from build123d import *

# Parameters (mm, degrees)
EXTRUDE_1_DEPTH          = 4
CUT_EXTRUDE_1_DEPTH      = 50.678969393496885
SKETCH_5_R               = 10
CUT_EXTRUDE_2_DEPTH      = 3.4
SKETCH_6_R               = 0.7
SKETCH_6_R_2             = 0.7000000000000005
CUT_EXTRUDE_3_DEPTH      = 50.24591353604885
SKETCH_8_R               = 4.25
CUT_EXTRUDE_5_DEPTH      = 50.24591353604885
CUT_EXTRUDE_7_DEPTH      = 50.193495504995376
CUT_EXTRUDE_7_DEPTH_BACK = 50.193495504995376
FILLET_1_R               = 1
CHAMFER_1_SIZE           = 1
CHAMFER_3_SIZE           = 1


with BuildPart() as part:
    # 草图1 → 凸台-拉伸1 (new, symmetric)
    with BuildSketch(Plane.XY):
        with BuildLine():
            Line((0.9523809523809523, 9.954545219222322), (42.57142857142857, 5.972727131533395))
            ThreePointArc((42.57142857142857, 5.972727131533395), (48, 0), (42.57142857142857, -5.972727131533395))
            Line((42.57142857142857, -5.972727131533395), (0.9523809523809523, -9.954545219222322))
            ThreePointArc((0.9523809523809523, -9.954545219222322), (-10.000000000000002, 1.22e-15), (0.9523809523809523, 9.954545219222322))
        make_face()
    extrude(amount=EXTRUDE_1_DEPTH, both=True)

    # 草图3 → 切除-拉伸1 (cut, through all)
    with BuildSketch(Plane.XY.offset(4)):
        with BuildLine():
            Line((38, 2.55), (42, 2.55))
            ThreePointArc((42, 2.55), (44.55, 0), (42, -2.55))
            Line((42, -2.55), (38, -2.55))
            ThreePointArc((38, -2.55), (35.45, 3.1e-16), (38, 2.55))
        make_face()
    extrude(amount=-CUT_EXTRUDE_1_DEPTH, mode=Mode.SUBTRACT)

    # 草图5 → 切除-拉伸2 (cut)
    with BuildSketch(Plane.XY.offset(4)):
        Circle(SKETCH_5_R)
    cut_extrude_2 = extrude(amount=-CUT_EXTRUDE_2_DEPTH, mode=Mode.SUBTRACT)

    # 镜向7: 切除-拉伸2 across plane
    add(cut_extrude_2.mirror(Plane.XY), mode=Mode.SUBTRACT)

    # 草图6 → 切除-拉伸3 (cut, through all)
    with BuildSketch(Plane.XY.offset(0.6000000000000003)):
        with Locations((0, 7)):
            Circle(SKETCH_6_R)
        with Locations((0, -7)):
            Circle(SKETCH_6_R)
        with Locations((7, -1.8e-15)):
            Circle(SKETCH_6_R_2)
        with Locations((-7, -1.8e-15)):
            Circle(SKETCH_6_R_2)
    extrude(amount=-CUT_EXTRUDE_3_DEPTH, mode=Mode.SUBTRACT)

    # 草图8 → 切除-拉伸5 (cut, through all)
    with BuildSketch(Plane.XY.offset(0.6000000000000003)):
        Circle(SKETCH_8_R)
    extrude(amount=-CUT_EXTRUDE_5_DEPTH, mode=Mode.SUBTRACT)

    # 草图10 → 切除-拉伸7 (cut, two sides: drawn at the far end of the back side and taken through both)
    with BuildSketch(Plane(origin=(0, 0, 0), x_dir=(1, 0, 0), z_dir=(0, 1, 0)).offset(-CUT_EXTRUDE_7_DEPTH_BACK)):
        Polygon((0.9523809523809523, 1.6000000000000003), (0.9523809523809523, 4), (20.952380952380953, 4.000000000000003), align=None)
        Polygon((0.9523809523809523, -2.4), (20.95238095238096, 6.07e-15), (48.00000000000001, 6.07e-15), (48.00000000000001, -4), (0.952380952380952, -4), align=None)
    extrude(amount=CUT_EXTRUDE_7_DEPTH + CUT_EXTRUDE_7_DEPTH_BACK, mode=Mode.SUBTRACT)

    # 圆角1
    fillet_1_edges = [part.edges().sort_by_distance(p)[0] for p in [
        (0.9523809523809526, 9.954545219222322, -1.0999999999999996),
        (0.9523809523809524, -9.954545219222322, -1.0999999999999996),
        (0.9523809523809526, 9.954545219222322, 1.5),
        (0.9523809523809524, -9.954545219222322, 1.5),
    ]]
    fillet(fillet_1_edges, radius=FILLET_1_R)

    # 倒角1
    chamfer_1_edges = [part.edges().sort_by_distance(p)[0] for p in [
        (31.761904761904763, 7.006906428907978, -4),
        (48, 1.33e-15, -4),
        (31.761904761904763, -7.006906428907978, -4),
        (48, 1.33e-15, -6.07e-15),
        (31.761904761904763, -7.006906428907977, -6.07e-15),
        (31.761904761904766, 7.006906428907978, -6.07e-15),
    ]]
    chamfer(chamfer_1_edges, length=CHAMFER_1_SIZE)

    # 倒角3
    # the kernel refuses this chamfer: 1 mm, written as the material it adds along each edge
    with BuildSketch(Plane(origin=(0, 0, -0.6000000000000001), x_dir=(0.6502681863563081, -0.7597047359421143, 0), z_dir=(-0.7597047359421143, -0.6502681863563081, 0))) as chamfer_3_piece_1:
        Polygon((10, -CHAMFER_3_SIZE), (9.999999999999998 - CHAMFER_3_SIZE, -2e-16), (9.999999999999998, 0), align=None)
    revolve(axis=Axis((0, 0, -0.6000000000000001), (0, 2e-17, 1)), revolution_arc=98.87634994501913)
    with BuildSketch(Plane(origin=(7.1529500499193945, 8.356752095363253, -0.6000000000000001), x_dir=(0.45453302112340566, -0.8907298876249914, 0), z_dir=(-0.8907298876249914, -0.45453302112340566, 0))) as chamfer_3_piece_2_section:
        Polygon((1.0000000000000004, -CHAMFER_3_SIZE), (1.0000000000000004 + CHAMFER_3_SIZE, 0), (1.0000000000000004, 0), align=None)
    chamfer_3_piece_2 = revolve(axis=Axis((7.1529500499193945, 8.356752095363253, -0.6000000000000001), (0, 0, 1)), revolution_arc=292.40328295994874, mode=Mode.PRIVATE)
    chamfer_3_piece_2 = split(chamfer_3_piece_2, bisect_by=Plane(origin=(6.105913725446883, 9.461491408882363, -0.9544569882762437), z_dir=(-0.09523809523809522, -0.995454521922232, 0)), keep=Keep.TOP, mode=Mode.PRIVATE)
    add(chamfer_3_piece_2)
    with BuildSketch(Plane(origin=(7.152950049919392, -8.356752095363255, -0.6000000000000001), x_dir=(0.4545330211234144, 0.8907298876249867, 0), z_dir=(-0.8907298876249867, 0.4545330211234144, 0))) as chamfer_3_piece_3_section:
        Polygon((1.0000000000000002 + CHAMFER_3_SIZE, 0), (0.9999999999999994, CHAMFER_3_SIZE), (1.0000000000000002, 0), align=None)
    chamfer_3_piece_3 = revolve(axis=Axis((7.152950049919392, -8.356752095363255, -0.6000000000000001), (0, 0, -1)), revolution_arc=292.40328295994846, mode=Mode.PRIVATE)
    chamfer_3_piece_3 = split(chamfer_3_piece_3, bisect_by=Plane(origin=(6.105912616149652, -9.46149151501213, -0.9544569410111913), z_dir=(-0.09523809523809522, 0.995454521922232, 0)), keep=Keep.TOP, mode=Mode.PRIVATE)
    add(chamfer_3_piece_3)


solid = part.part
Geometry check sheet. Reference: the model listing, model coordinates, mm. A direction names the side the tool comes from. Give positions to 0.01 mm unless a question says otherwise; leave off trailing zeros. Order: outer loops, then holes, each group sorted by start corner. A loop starts at its lowest first (then second) coordinate and runs counter-clockwise, first axis right, second up.
1. Depth check by flat-ended pin: pin 1 (4 mm diameter, centred on x = -4, y = 7, fed in from -Z); pin 2 (3 mm diameter, centred on x = 40, z = -2, fed in from -Y); pin 3 (11.5 mm diameter, centred on x = 33.5, y = -1.5, fed in from +Z). Enter the tip coordinate at first touch or a pass-through.
Completed:
pin 1: stops at z = -0.6
pin 2: stops at y = -6.36
pin 3: stops at z = 0
2. Draft check along Y on faces 1 (the face through (34.3, 6.27, -0.51)), 2 (the face through (48, 0, -2)), 3 (the face through (6.3, 0, 0)). Enter one of: pulls with the +Y half, pulls with the -Y half, needs draft (parallel to the pull), parting line crosses it, or undercut.
Completed:
face 1: pulls with the +Y half
face 2: parting line crosses it
face 3: undercut
3. Access from +Z, -Z, +X, -X, +Y, -Y to the whole of each face (thin tool, end or side, straight path). Record for faces 4 (the face through (10, 0, -2)), 5 (the face through (40, -2.55, -2)), 6 (the face through (31, 0, 0)).
Completed:
face 4: -Z, -X
face 5: +Z, -Z
face 6: +Z, +X, +Y, -Y
4. Sectioned sample at B-B (x = -7). Record the boundary of the cut face in (y, z).
Completed:
outline: (-7.14, -0.6) - (-0.7, -0.6) - (-0.7, 0.6) - (-7.14, 0.6) - close; (0.7, -0.6) - (7.14, -0.6) - (7.14, 0.6) - (0.7, 0.6) - close
5. Sectioned sample at A-A (x = 0). Record the boundary of the cut face in (y, z), then the cut area to 3 significant figures.
Completed:
outline: (-10, -0.6) - (-7.7, -0.6) - (-7.7, 0.6) - (-10, 0.6) - close; (-6.3, -0.6) - (-4.25, -0.6) - (-4.25, 0.6) - (-6.3, 0.6) - close; (4.25, -0.6) - (6.3, -0.6) - (6.3, 0.6) - (4.25, 0.6) - close; (7.7, -0.6) - (10, -0.6) - (10, 0.6) - (7.7, 0.6) - close
area: 10.4 mm2
6. Scan lines: line 1 (Y direction, x = 0, z = 0.3); line 2 (Y direction, x = 0.5, z = 0.45); line 3 (Z direction, x = 23.5, y = 0.25). Record each from-to range of solid material in increasing order.
Completed:
line 1: y = -10 to -7.7, -6.3 to -4.25, 4.25 to 6.3, 7.7 to 10
line 2: y = -9.99 to -7.49, -6.51 to -4.22, 4.22 to 6.51, 7.49 to 9.99
line 3: z = -4 to 0
7. Sectioned sample at C-C (y = 0). State how many separate pieces and enclosed holes the cut face has, then the cut area to 3 significant figures.
Completed:
separate pieces: 5
enclosed holes: 0
area: 126 mm2
8. Sectioned sample at D-D (x = 15). Record the boundary of the cut face in (y, z).
Completed:
outline: (-8.61, -3) - (-8.32, -3.29) - (8.32, -3.29) - (8.61, -3) - (8.61, 0.71) - (-8.61, 0.71) - close
